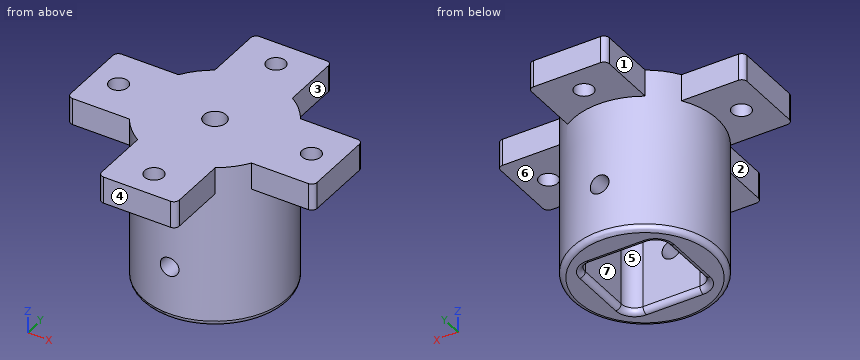
```python
from build123d import *
from build123d.topology import SkipClean

# Parameters (mm, degrees)
SKETCH1_R               = 13.5
SKETCH1_R_2             = 2.1
BOSS_EXTRUDE1_DEPTH     = 5.5
SKETCH2_R               = 13.5
SKETCH2_R_2             = 2.1
BOSS_EXTRUDE2_DEPTH     = 5
SKETCH4_W               = 14.5
SKETCH4_H               = 15
SKETCH4_W_2             = 15
SKETCH4_H_2             = 14.5
BOSS_EXTRUDE4_DEPTH     = 5
CUT_EXTRUDE1_REACH      = 34.989
SKETCH5_R               = 1.75
BOSS_EXTRUDE5_START     = 20
SKETCH6_R               = 13.5
BOSS_EXTRUDE5_DEPTH     = 20
CUT_EXTRUDE2_DEPTH      = 39.183766184
CUT_EXTRUDE2_DEPTH_BACK = 39.183766184
SKETCH7_R               = 1.75
FILLET5_R               = 1
FILLET6_R               = 1


with BuildPart() as part:
    # Sketch1 → Boss-Extrude1 (new body)
    with BuildSketch(Plane.XY):
        Circle(SKETCH1_R)
        Circle(SKETCH1_R_2, mode=Mode.SUBTRACT)
    extrude(amount=BOSS_EXTRUDE1_DEPTH)

    # Sketch2 → Boss-Extrude2 (add)
    with BuildSketch(Plane.XY.offset(5.5)):
        Circle(SKETCH2_R)
        Circle(SKETCH2_R_2, mode=Mode.SUBTRACT)
    extrude(amount=BOSS_EXTRUDE2_DEPTH)

    # Sketch4 → Boss-Extrude4 (add)
    with BuildSketch(Plane.XY.offset(10.5)):
        with Locations((0, 15.5)):
            Rectangle(SKETCH4_W, SKETCH4_H)
        with Locations((15.5, 0)):
            Rectangle(SKETCH4_W_2, SKETCH4_H_2)
        with Locations((-15.5, 0)):
            Rectangle(SKETCH4_W_2, SKETCH4_H_2)
        with Locations((0, -15.5)):
            Rectangle(SKETCH4_W, SKETCH4_H)
    extrude(amount=-BOSS_EXTRUDE4_DEPTH)

    # Sketch5 → Cut-Extrude1 (cut, up to next)
    with BuildSketch(Plane(origin=(0, 0, 5.5), x_dir=(-1, 0, 0), z_dir=(0, 0, -1)), mode=Mode.PRIVATE) as cut_extrude1_sk1:
        with Locations((18, 0)):
            Circle(SKETCH5_R)
    cut_extrude1_tool1 = extrude(cut_extrude1_sk1.sketch, amount=-CUT_EXTRUDE1_REACH, mode=Mode.PRIVATE) & part.part
    # Sketch5 → Cut-Extrude1 (cut, up to next)
    with BuildSketch(Plane(origin=(0, 0, 5.5), x_dir=(-1, 0, 0), z_dir=(0, 0, -1)), mode=Mode.PRIVATE) as cut_extrude1_sk2:
        with Locations((-18, 0)):
            Circle(SKETCH5_R)
    cut_extrude1_tool2 = extrude(cut_extrude1_sk2.sketch, amount=-CUT_EXTRUDE1_REACH, mode=Mode.PRIVATE) & part.part
    # Sketch5 → Cut-Extrude1 (cut, up to next)
    with BuildSketch(Plane(origin=(0, 0, 5.5), x_dir=(-1, 0, 0), z_dir=(0, 0, -1)), mode=Mode.PRIVATE) as cut_extrude1_sk3:
        with Locations((0, 18)):
            Circle(SKETCH5_R)
    cut_extrude1_tool3 = extrude(cut_extrude1_sk3.sketch, amount=-CUT_EXTRUDE1_REACH, mode=Mode.PRIVATE) & part.part
    # Sketch5 → Cut-Extrude1 (cut, up to next)
    with BuildSketch(Plane(origin=(0, 0, 5.5), x_dir=(-1, 0, 0), z_dir=(0, 0, -1)), mode=Mode.PRIVATE) as cut_extrude1_sk4:
        with Locations((0, -18)):
            Circle(SKETCH5_R)
    cut_extrude1_tool4 = extrude(cut_extrude1_sk4.sketch, amount=-CUT_EXTRUDE1_REACH, mode=Mode.PRIVATE) & part.part
    add(cut_extrude1_tool1.solids().sort_by_distance((-18, 0, 5.5))[0], mode=Mode.SUBTRACT)
    add(cut_extrude1_tool2.solids().sort_by_distance((18, 0, 5.5))[0], mode=Mode.SUBTRACT)
    add(cut_extrude1_tool3.solids().sort_by_distance((0, 18, 5.5))[0], mode=Mode.SUBTRACT)
    add(cut_extrude1_tool4.solids().sort_by_distance((0, -18, 5.5))[0], mode=Mode.SUBTRACT)

    # Sketch6 → Boss-Extrude5 (add)
    with SkipClean():  # the faces are left unmerged after this step: merging them gives an invalid solid
        with BuildSketch(Plane(origin=(0, 0, 0), x_dir=(-1, 0, 0), z_dir=(0, 0, -1)).offset(BOSS_EXTRUDE5_START)):
            Circle(SKETCH6_R)
            with BuildLine():
                Line((-5.3, 7.8), (5.3, 7.8))
                ThreePointArc((5.3, 7.8), (7.067766953, 7.067766953), (7.8, 5.3))
                Line((7.8, 5.3), (7.8, -5.3))
                ThreePointArc((7.8, -5.3), (7.067766953, -7.067766953), (5.3, -7.8))
                Line((5.3, -7.8), (-5.3, -7.8))
                ThreePointArc((-5.3, -7.8), (-7.067766953, -7.067766953), (-7.8, -5.3))
                Line((-7.8, -5.3), (-7.8, 5.3))
                ThreePointArc((-7.8, 5.3), (-7.067766953, 7.067766953), (-5.3, 7.8))
            make_face(mode=Mode.SUBTRACT)
        extrude(amount=-BOSS_EXTRUDE5_DEPTH)

    # Sketch7 → Cut-Extrude2 (cut, two sides: drawn at the far end of the back side and taken through both)
    with SkipClean():  # the faces are left unmerged after this step: merging them gives an invalid solid
        with BuildSketch(Plane(origin=(0, 0, 0), x_dir=(1, 0, 0), z_dir=(0, 1, 0)).offset(-CUT_EXTRUDE2_DEPTH_BACK)):
            with Locations(Location((0, 10, 0), (0, 0, 270))):
                Circle(SKETCH7_R)
        extrude(amount=CUT_EXTRUDE2_DEPTH + CUT_EXTRUDE2_DEPTH_BACK, mode=Mode.SUBTRACT)

    # Fillet5
    fillet5_edges = [part.edges().sort_by_distance(p)[0] for p in [
        (13.5, 0, -20),
        (7.067766953, -7.067766953, -20),
        (0, -7.8, -20),
        (-7.067766953, -7.067766953, -20),
        (-7.8, 0, -20),
        (-7.067766953, 7.067766953, -20),
        (0, 7.8, -20),
        (7.067766953, 7.067766953, -20),
        (7.8, 0, -20),
    ]]
    fillet(fillet5_edges, radius=FILLET5_R)

    # Fillet6
    fillet6_edges = [part.edges().sort_by_distance(p)[0] for p in [
        (7.25, 23, 8),
        (-7.25, 23, 8),
        (23, -7.25, 8),
        (23, 7.25, 8),
        (-23, 7.25, 8),
        (-23, -7.25, 8),
        (-7.25, -23, 8),
        (7.25, -23, 8),
    ]]
    fillet(fillet6_edges, radius=FILLET6_R)


solid = part.part
```
Here's how the part is built. I have some questions about the finished solid (model axes, mm). Face numbers are marked on the shaded views. A direction names the side the tool comes from. Give positions to 0.01 mm unless a question says otherwise; leave off trailing zeros. Loops run counter-clockwise (first coordinate to the right, second up) from the corner with the lowest first, then second, coordinate; pieces in that order, holes last. Notation, with made-up numbers: M 75.25,69 L 80.25,69 A33 ccw 80.25,100 Z; hole C 68,81.25 d3. An arc over 180 degrees is marked long. Return JSON: item names as keys, results as strings.
Item 1: Thinking about a two-plate mould opening in Y: for the marked faces 4, 5, 6 and 7, which applies, released by +Y, released by -Y, zero draft, split by the parting line, or undercut?
A:
{"face 4": "released by -Y", "face 5": "undercut", "face 6": "zero draft", "face 7": "undercut"}
Item 2: Imagine slicing it at C-C on z = -5.5. List the corners of the cut face in (x, y) for me, then the cut area to 3 significant figures.
A:
{"outline": "C 0,0 d27; hole M -7.8,-5.3 A2.5 ccw -5.3,-7.8 L 5.3,-7.8 A2.5 ccw 7.8,-5.3 L 7.8,5.3 A2.5 ccw 5.3,7.8 L -5.3,7.8 A2.5 ccw -7.8,5.3 Z", "area": "335 mm^2"}
Item 3: On a 3-axis mill with a long thin cutter (end or side, diameter ignored), from which of +Z, -Z, +X, -X, +Y, -Y can I reach the whole of each face in a straight line? I mean the marked faces 1, 2 and 3. Say none if no direction works.
A:
{"face 1": "+Z, -Z, -X, +Y", "face 2": "+Z, -Z, -X, -Y", "face 3": "+Z, -Z, +X, +Y"}
Item 4: Imagine slicing it at D-D on y = 0. List the corners of the cut face in (x, z) for me.
A:
{"outline": "M -23,5.5 L -19.75,5.5 L -19.75,10.5 L -23,10.5 Z; M -16.25,5.5 L -13.5,5.5 L -13.5,-19 A1 ccw -12.5,-20 L -8.8,-20 A1 ccw -7.8,-19 L -7.8,0 L -2.1,0 L -2.1,10.5 L -16.25,10.5 Z; M 2.1,0 L 7.8,0 L 7.8,-19 A1 ccw 8.8,-20 L 12.5,-20 A1 ccw 13.5,-19 L 13.5,5.5 L 16.25,5.5 L 16.25,10.5 L 2.1,10.5 Z; M 19.75,5.5 L 23,5.5 L 23,10.5 L 19.75,10.5 Z"}
Item 5: I'm going to push flat-ended pins straight in: pin 1 Ø8 at (y, z) = (-6.5, -1.5) entering from -X; pin 2 Ø8.5 at (y, z) = (-0.5, -9) entering from -X; pin 3 Ø5.5 at (x, z) = (-15, 8.5) entering from -Y. Where does each tip first touch, or does it pass through?
A:
{"pin 1": "stops at x = -13.27", "pin 2": "stops at x = -13.5", "pin 3": "stops at y = -7.25"}
Item 6: Imagine slicing it at A-A on y = 18. List the corners of the cut face in (x, z) for me.
A:
{"outline": "M -7.25,5.5 L -1.75,5.5 L -1.75,10.5 L -7.25,10.5 Z; M 1.75,5.5 L 7.25,5.5 L 7.25,10.5 L 1.75,10.5 Z"}
Item 7: Please list where these lines run through material, in increasing order: line 1 (Y direction, x = -18, z = 8.15); line 2 (Z direction, x = 3.5, y = 21); line 3 (Z direction, x = 1.5, y = -6).
A:
{"line 1": "y = -7.25 to -1.75, 1.75 to 7.25", "line 2": "z = 5.5 to 10.5", "line 3": "z = 0 to 10.5"}
